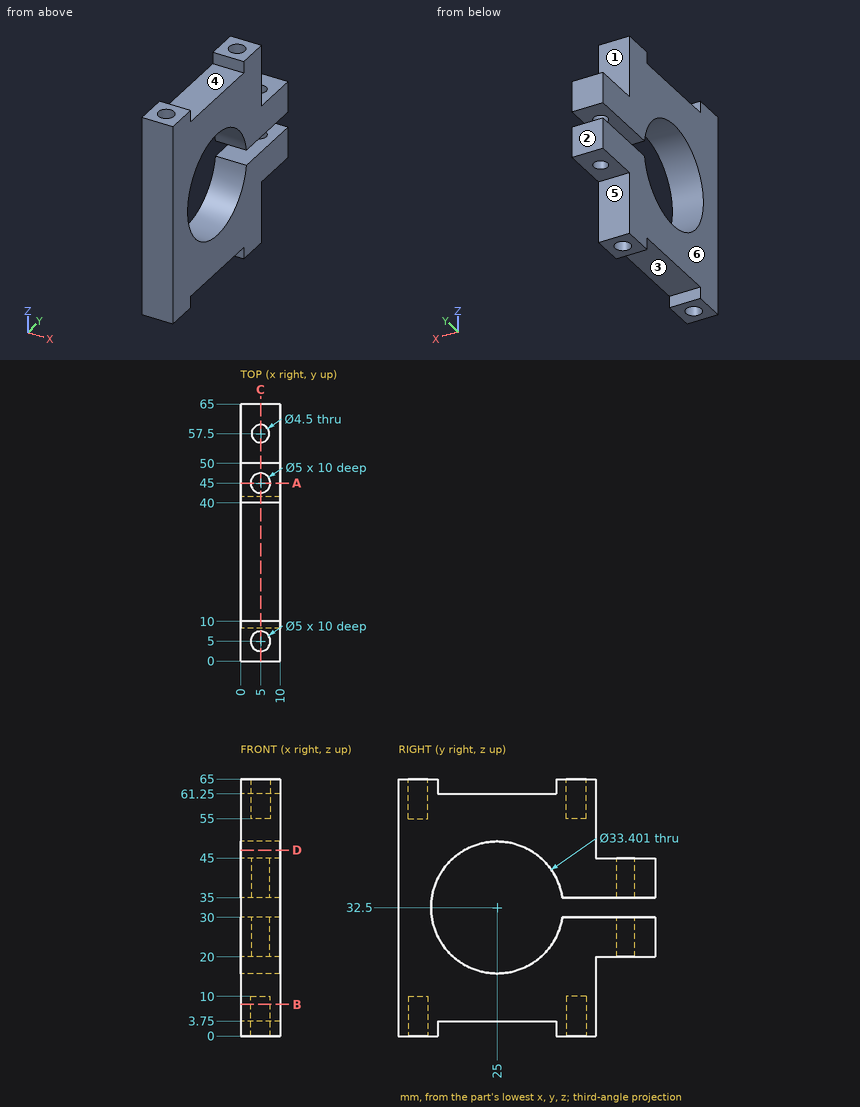
Design review of the part shown in the three views and the two pictorial views. Dimensions are in mm from the part's minimum x, y and z. A direction names the side the tool comes from. Give positions to 0.01 mm unless a question says otherwise; leave off trailing zeros. Write each loop counter-clockwise with the first axis right and the second up, starting at its lowest first coordinate (ties: lowest second). Pieces come first, ordered by that corner, then holes. Notation, with made-up numbers: (26.5, 19.25) - (74.5, 19.25) arc R28 cw to (74.5, 42.25) - close; hole circle Ø11 at (89, 14.25). An arc over 180 degrees is marked (long way). Return JSON: item names as keys, results as strings. Group by question number.
(1) We need section B-B, the plane z = 8. Give the boundary of the cut face in (x, y).
(2) We need section D-D, the plane z = 47. Give the boundary of the cut face in (x, y).
(3) Mouldability with a two-part tool opening along Y and no side actions: class the marked faces 3, 4, 5 and 6 as +Y half, -Y half, draft (parallel to the pull), parting line (faces both ways), or undercut.
(4) Machinability: for the marked faces 1 and 2, which of the approach directions +Z, -Z, +X, -X, +Y, -Y give a long, thin tool a straight path to every point of the face, cutting with its end or side? Answer none if there is none.
(5) Insertion check: pin 1 (5 mm diameter, centred on x = 3.5, y = 27, fed in from +Z); pin 2 (1.5 mm diameter, centred on x = 7.5, y = 35, fed in from -Z); pin 3 (2 mm diameter, centred on x = 7.5, z = 33, fed in from +Y). Each pin has a flat end and moves straight along its axis. Give the tip position at first contact, or say it passes through.
(6) We need section A-A, the plane y = 45. Give the boundary of the cut face in (x, z), then the cut area to 3 significant figures.
(7) We need section C-C, the plane x = 5. Give the number of separate pieces and of enclosed holes in the cut face, then the cut area to 3 significant figures.
(8) To check wall thickness, follow probe 1 along X at (y, z) = (5, 60); probe 2 along Y at (x, z) = (5, 3); probe 3 along Z at (x, y) = (3.5, 55.5). State the ranges of each line that lie inside material, in increasing order.
Reported:
{
 "1": {"outline": "(0, 0) - (10, 0) - (10, 50) - (0, 50) - close; hole circle Ø5 at (5, 5); hole circle Ø5 at (5, 45)"},
 "2": {"outline": "(0, 0) - (10, 0) - (10, 16.71) - (0, 16.71) - close; (0, 33.29) - (10, 33.29) - (10, 50) - (0, 50) - close"},
 "3": {"face 3": "undercut", "face 4": "undercut", "face 5": "+Y half", "face 6": "draft"},
 "4": {"face 1": "+Z, +X, -X, +Y", "face 2": "+Z, -Z, +X, -X, +Y"},
 "5": {"pin 1": "stops at z = 61.25", "pin 2": "stops at z = 3.75", "pin 3": "stops at y = 8.37"},
 "6": {"outline": "(0, 0) - (2.5, 0) - (2.5, 10) - (7.5, 10) - (7.5, 0) - (10, 0) - (10, 30) - (0, 30) - close; (0, 35) - (10, 35) - (10, 65) - (7.5, 65) - (7.5, 55) - (2.5, 55) - (2.5, 65) - (0, 65) - close", "area": "500 mm2"},
 "7": {"separate pieces": "3", "enclosed holes": "0", "area": "2,120 mm2"},
 "8": {"probe 1": "x = 0 to 2.5, 7.5 to 10", "probe 2": "y = 0 to 2.5, 7.5 to 10, 40 to 42.5, 47.5 to 50", "probe 3": "z = 20 to 30, 35 to 45"}
}
